from build123d import *

# Parameters (mm, degrees)
CROQUIS1_W              = 30
CROQUIS1_H              = 75
CROQUIS1_R              = 2.05
CROQUIS1_R_2            = 2.55
SALIENTE_EXTRUIR1_DEPTH = 5
REDONDEO1_R             = 4
CROQUIS4_R              = 4.05
CORTAR_EXTRUIR1_DEPTH   = 2.8


with BuildPart() as part:
    # Croquis1 → Saliente-Extruir1 (new body)
    with BuildSketch(Plane.XY):
        with Locations((15, 37.5)):
            Rectangle(CROQUIS1_W, CROQUIS1_H)
        with Locations((5, 66.8)):
            Circle(CROQUIS1_R, mode=Mode.SUBTRACT)
        with Locations((25, 66.8)):
            Circle(CROQUIS1_R, mode=Mode.SUBTRACT)
        with Locations((25, 46.8)):
            Circle(CROQUIS1_R, mode=Mode.SUBTRACT)
        with Locations((5, 46.8)):
            Circle(CROQUIS1_R, mode=Mode.SUBTRACT)
        with Locations((15, 11.08)):
            Circle(CROQUIS1_R_2, mode=Mode.SUBTRACT)
    extrude(amount=SALIENTE_EXTRUIR1_DEPTH)

    # Redondeo1
    redondeo1_edges = [part.edges().sort_by_distance(p)[0] for p in [
        (0, 75, 2.5),
        (30, 75, 2.5),
        (30, 0, 2.5),
        (0, 0, 2.5),
    ]]
    fillet(redondeo1_edges, radius=REDONDEO1_R)

    # Croquis4 → Cortar-Extruir1 (cut)
    with BuildSketch(Plane.XY.offset(5)):
        with Locations((5, 66.8)):
            Circle(CROQUIS4_R)
        with Locations((5, 46.8)):
            Circle(CROQUIS4_R)
        with Locations((25, 46.8)):
            Circle(CROQUIS4_R)
        with Locations((25, 66.8)):
            Circle(CROQUIS4_R)
    extrude(amount=-CORTAR_EXTRUIR1_DEPTH, mode=Mode.SUBTRACT)


solid = part.part
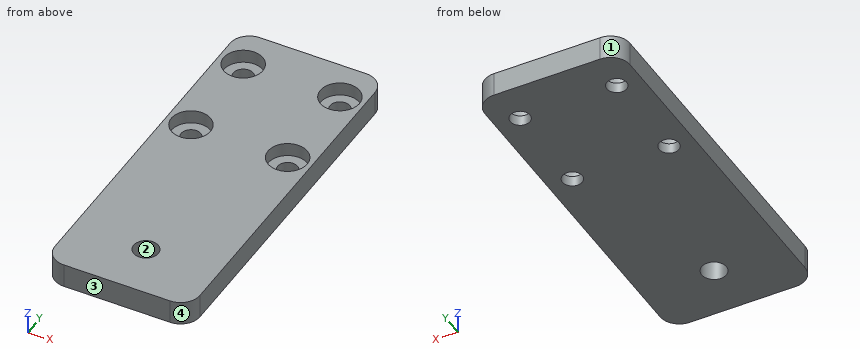
Design review of the part built by this model. Coordinates are the model's own, in mm. Face numbers are marked on the shaded views. Round coordinates to 2 decimals unless told otherwise and drop trailing zeros. Write each loop counter-clockwise with the first axis right and the second up, starting at its lowest first coordinate (ties: lowest second). Pieces come first, ordered by that corner, then holes. Notation, with made-up numbers: (65.25, 58) -> (101.25, 58) arc R24 cw to (101.25, 82) -> close; hole circle Ø9 at (32.25, 86.25). An arc over 180 degrees is marked (long way). One line per question, with ' | ' between items.
(1) Take a section at C-C, the plane y = 11.08. State the section outline as (x, z) points.
Result sheet:
outline: (0, 0) -> (12.45, 0) -> (12.45, 5) -> (0, 5) -> close; (17.55, 0) -> (30, 0) -> (30, 5) -> (17.55, 5) -> close
(2) Draft analysis for pull direction X (two halves, no side actions). For the marked faces 1, 2, 3 and 4, state which applies: released by +X, released by -X, zero draft, split by the parting line, or undercut.
Result sheet:
face 1: released by -X | face 2: undercut | face 3: zero draft | face 4: released by +X
(3) Wall thickness on line 1 (X direction, y = 66.8, z = 0.75); line 2 (Y direction, x = 5, z = 3.15); line 3 (X direction, y = 66.5, z = 2.5): over which ranges is each line inside the solid? List them lowest first. Write a range as [from, to].
Result sheet:
line 1: [0, 2.95], [7.05, 22.95], [27.05, 30] | line 2: [0, 42.75], [50.85, 62.75], [70.85, 75] | line 3: [0, 0.96], [9.04, 20.96], [29.04, 30]
(4) Take a section at A-A, the plane x = 25. State the section outline as (y, z) points.
Result sheet:
outline: (0, 0) -> (44.75, 0) -> (44.75, 2.2) -> (42.75, 2.2) -> (42.75, 5) -> (0, 5) -> close; (48.85, 0) -> (64.75, 0) -> (64.75, 2.2) -> (62.75, 2.2) -> (62.75, 5) -> (50.85, 5) -> (50.85, 2.2) -> (48.85, 2.2) -> close; (68.85, 0) -> (75, 0) -> (75, 5) -> (70.85, 5) -> (70.85, 2.2) -> (68.85, 2.2) -> close
(5) Take a section at D-D, the plane z = 1.15. State the section outline as (x, y) points, and give its area (3 significant figures).
Result sheet:
outline: (0, 4) arc R4 ccw to (4, 0) -> (26, 0) arc R4 ccw to (30, 4) -> (30, 71) arc R4 ccw to (26, 75) -> (4, 75) arc R4 ccw to (0, 71) -> close; hole circle Ø4.1 at (5, 46.8); hole circle Ø4.1 at (5, 66.8); hole circle Ø5.1 at (15, 11.08); hole circle Ø4.1 at (25, 46.8); hole circle Ø4.1 at (25, 66.8) | area: 2,160 mm2
(6) Take a section at B-B, the plane y = 66.8. State the section outline as (x, z) points, and give its area (3 significant figures).
Result sheet:
outline: (0, 0) -> (2.95, 0) -> (2.95, 2.2) -> (0.95, 2.2) -> (0.95, 5) -> (0, 5) -> close; (7.05, 0) -> (22.95, 0) -> (22.95, 2.2) -> (20.95, 2.2) -> (20.95, 5) -> (9.05, 5) -> (9.05, 2.2) -> (7.05, 2.2) -> close; (27.05, 0) -> (30, 0) -> (30, 5) -> (29.05, 5) -> (29.05, 2.2) -> (27.05, 2.2) -> close | area: 86.6 mm2
(7) Insertion check: P1, Ø6, axis at x = 15, y = 11.08, coming from the +Z side; P2, Ø2.5, axis at x = 5, y = 48, coming from the +Z side; P3, Ø3.5, axis at x = 5, y = 46.8, coming from the +Z side. Each pin has a flat end and moves straight along its axis. Give the tip position at first contact, or say it passes through.
Result sheet:
P1: z = 5 | P2: z = 2.2 | P3: through
